Autodesk Inventor part; units mm, degrees
ref_plane "Work Plane2" through (15.7, -2, 0) normal (1, 0, 0) x (0, 1, 0)
ref_plane "XZ Plane" through (0, 0, 0) normal (0, 1, 0) x (-1, 0, 0)
ref_plane "XY Plane" through (0, 0, 0) normal (0, 0, 1) x (1, 0, 0)
sketch "Sketch1" plane through (0, 0, 0) normal (0, 0, 1) x (1, 0, 0)
  line L0 (0, 0) -> (12.7, 0)
  arc A0 (13.2, -0.5) -> (12.7, 0) centre (12.7, -0.5) ccw
  line L1 (13.2, -0.5) -> (13.2, -1.5)
  arc A1 (13.2, -1.5) -> (13.7, -2) centre (13.7, -1.5) ccw
  line L2 (13.7, -2) -> (15.7, -2)
  dimension "d0" = 0.5
  dimension "d1" = 2
  dimension "d2" = 90
  dimension "d3" = 12.7
  dimension "d5" = 2
ref_plane "Work Plane2" through (15.7, -2, 0) normal (1, 0, 0) x (0, 1, 0)
sketch "Sketch3" plane through (15.7, -2, 0) normal (1, 0, 0) x (0, 1, 0)
  circle A0 centre (0, 0) radius 0.4
  point P0 (2, 0)
  dimension "d6" = 0.8
sweep "Sweep1" add profiles "Sketch3" path "Sketch1"
mirror "Mirror1" about plane through (0, 0, 0) normal (-1, 0, 0) of "Sweep1"
properties part number "rotobot pushrod"
Input: part model. Units: mm. Frame: model coordinates. Coordinates: 2 decimals unless noted, no trailing zeros. Write each loop counter-clockwise with the first axis right and the second up, starting at its lowest first coordinate (ties: lowest second). Pieces come first, ordered by that corner, then holes. Notation, with made-up numbers: (82, 88.5) - (115, 88.5) arc R19 cw to (115, 122.5) - close; hole circle Ø4 at (66.25, -21). An arc over 180 degrees is marked (long way). Put each result on its own line as item: value. Start each with the question number.
1) Cut plane B-B (x = 11). Return the cut outline in (y, z), plus the area to 3 significant figures.
2) Cut plane A-A (z = 0). Return the cut outline in (x, y).
3) Ray query, L1, parallel to X at y = -1.45, z = -0.05; L2, parallel to X at y = -2.25, z = -0.2; L3, parallel to Z at x = -3, y = -0.05. Return the intervals inside material, ascending.
Resolved:
1. outline: circle Ø0.8 at (0, 0)
1. area: 0.503 mm2
2. outline: (-15.7, -2.4) - (-13.7, -2.4) arc R0.9 ccw to (-12.8, -1.5) - (-12.8, -0.5) arc R0.1 cw to (-12.7, -0.4) - (12.7, -0.4) arc R0.1 cw to (12.8, -0.5) - (12.8, -1.5) arc R0.9 ccw to (13.7, -2.4) - (15.7, -2.4) - (15.7, -1.6) - (13.7, -1.6) arc R0.1 cw to (13.6, -1.5) - (13.6, -0.5) arc R0.9 ccw to (12.7, 0.4) - (-12.7, 0.4) arc R0.9 ccw to (-13.6, -0.5) - (-13.6, -1.5) arc R0.1 cw to (-13.7, -1.6) - (-15.7, -1.6) - close
3. L1: x = -13.6 to -12.8, 12.8 to 13.6
3. L2: x = -15.7 to -13.31, 13.31 to 15.7
3. L3: z = -0.4 to 0.4
